The listing builds one solid part. Answer for the finished solid, in the listing's coordinates (mm). A direction names the side the tool comes from. Coordinates: 2 decimals unless noted, no trailing zeros. Loops run counter-clockwise (first coordinate to the right, second up) from the corner with the lowest first, then second, coordinate; pieces in that order, holes last. Notation, with made-up numbers: (-24, 34) - (15, 34) arc R27 cw to (15, 50) - close; hole circle Ø7 at (7.5, 21.5). An arc over 180 degrees is marked (long way). Use one line per item in the form item = value. Start each with the question number.
```python
from build123d import *

# Parameters (mm, degrees)
SKETCH_1_W          = 10
SKETCH_1_H          = 10
SKETCH_1_W_2        = 8
SKETCH_1_H_2        = 8
EXTRUDE_1_DEPTH     = 250
SKETCH_2_R          = 1.6
CUT_EXTRUDE_1_DEPTH = 251.249875125
SKETCH_3_R          = 1.6
CUT_EXTRUDE_2_DEPTH = 60


with BuildPart() as part:
    # ｽｹｯﾁ1 → ﾎﾞｽ - 押し出し1 (new body)
    with BuildSketch(Plane.XY):
        Rectangle(SKETCH_1_W, SKETCH_1_H)
        Rectangle(SKETCH_1_W_2, SKETCH_1_H_2, mode=Mode.SUBTRACT)
    extrude(amount=EXTRUDE_1_DEPTH)

    # ｽｹｯﾁ2 → ｶｯﾄ - 押し出し1 (cut, through all)
    with BuildSketch(Plane(origin=(0, 5, 0), x_dir=(1, 0, 0), z_dir=(0, 1, 0))):
        with Locations(Location((0, -215, 0), (0, 0, 180))):
            Circle(SKETCH_2_R)
        with Locations(Location((0, -245, 0), (0, 0, 180))):
            Circle(SKETCH_2_R)
        with Locations(Location((0, -230, 0), (0, 0, 180))):
            Circle(SKETCH_2_R)
    extrude(amount=-CUT_EXTRUDE_1_DEPTH, mode=Mode.SUBTRACT)

    # ｽｹｯﾁ3 → ｶｯﾄ - 押し出し2 (cut)
    with BuildSketch(Plane(origin=(5, 0, 0), x_dir=(0, 0, -1), z_dir=(1, 0, 0))):
        with Locations((-5, 0)):
            Circle(SKETCH_3_R)
    extrude(amount=-CUT_EXTRUDE_2_DEPTH, mode=Mode.SUBTRACT)


solid = part.part
```
(1) This flat-tipped pin is pushed along its axis until it touches: pin 1 Ø2.5 at (x, z) = (0, 215) entering from -Y. Where does it stop, or does it pass through?
(2) A cutting plane is placed at B-B (y = 0). Determine the outline of the cut face in (x, z).
(3) For faces 4 (the face through (0, -5, 123)), 5 (the face through (4, 0, 123)), determine the directions among +Z, -Z, +X, -X, +Y, -Y from which every point of the face is accessible in a straight line to the end or side of a thin tool.
(4) A cutting plane is placed at C-C (x = 0). State how many separate pieces and enclosed holes the cut face has, then the cut area to 3 significant figures.
(5) A cutting plane is placed at A-A (z = 195). Determine the outline of the cut face in (x, y).
(6) Find the intervals of material crossed by probe 1 along Z at (x, y) = (0, -4.3); probe 2 along X at (y, z) = (4.35, 215); probe 3 along Y at (x, z) = (3.5, 225), in increasing order. Write a range as from..to.
(7) Determine the mould class of faces 1 (the face through (5, 0, 123)), 2 (the face through (0, 4, 123)), 3 (the face through (-4.5, 0.1, 0)) for opening direction X: +X half, -X half, draft (parallel to the pull), parting line (faces both ways), or undercut.
Evaluation:
q1.pin_1 = through
q2.outline = (-5, 0) - (-4, 0) - (-4, 3.4) - (-5, 3.4) - close; (-5, 6.6) - (-4, 6.6) - (-4, 250) - (-5, 250) - close; (4, 0) - (5, 0) - (5, 3.4) - (4, 3.4) - close; (4, 6.6) - (5, 6.6) - (5, 250) - (4, 250) - close
q3.face_4 = +Z, -Z, +X, -X, -Y
q3.face_5 = +Z, -Z
q4.separate_pieces = 8
q4.enclosed_holes = 0
q4.area = 481 mm^2
q5.outline = (-5, -5) - (5, -5) - (5, 5) - (-5, 5) - close; hole (-4, -4) - (4, -4) - (4, 4) - (-4, 4) - close
q6.probe_1 = 0..213.4, 216.6..228.4, 231.6..243.4, 246.6..250
q6.probe_2 = -5..-1.6, 1.6..5
q6.probe_3 = -5..-4, 4..5
q7.face_1 = +X half
q7.face_2 = undercut
q7.face_3 = draft
